from build123d import *

# Parameters (mm, degrees)
SKETCH1_W                      = 19
SKETCH1_H                      = 19
SKETCH1_R                      = 6.5
BOSS_EXTRUDE1_DEPTH            = 4
CUT_EXTRUDE1_REACH             = 16.018
SKETCH2_R                      = 1.5
CUT_EXTRUDE1_DIRECTION_2_REACH = 16.018
SKETCH5_W                      = 4
SKETCH5_H                      = 5
BOSS_EXTRUDE3_DEPTH            = 8
CUT_EXTRUDE2_REACH             = 22.31
SKETCH7_R                      = 1.5
CUT_EXTRUDE2_DIRECTION_2_REACH = 22.31


with BuildPart() as part:
    # Sketch1 → Boss-Extrude1 (new body)
    with BuildSketch(Plane.XY):
        Rectangle(SKETCH1_W, SKETCH1_H)
        Circle(SKETCH1_R, mode=Mode.SUBTRACT)
    extrude(amount=BOSS_EXTRUDE1_DEPTH)

    # Sketch2 → Cut-Extrude1 (cut, up to next)
    with BuildSketch(Plane(origin=(0, 0, 0), x_dir=(1, 0, 0), z_dir=(0, 1, 0)), mode=Mode.PRIVATE) as cut_extrude1_sk1:
        with Locations(Location((0, -2, 0), (0, 0, 90))):
            Circle(SKETCH2_R)
    cut_extrude1_tool1 = extrude(cut_extrude1_sk1.sketch, amount=CUT_EXTRUDE1_REACH, mode=Mode.PRIVATE) & part.part
    add(cut_extrude1_tool1.solids().sort_by_distance((0, 0, 2))[0], mode=Mode.SUBTRACT)

    # Sketch2 → Cut-Extrude1 direction 2 (cut, up to next)
    with BuildSketch(Plane(origin=(0, 0, 0), x_dir=(1, 0, 0), z_dir=(0, 1, 0)), mode=Mode.PRIVATE) as cut_extrude1_direction_2_sk1:
        with Locations(Location((0, -2, 0), (0, 0, 90))):
            Circle(SKETCH2_R)
    cut_extrude1_direction_2_tool1 = extrude(cut_extrude1_direction_2_sk1.sketch, amount=-CUT_EXTRUDE1_DIRECTION_2_REACH, mode=Mode.PRIVATE) & part.part
    add(cut_extrude1_direction_2_tool1.solids().sort_by_distance((0, 0, 2))[0], mode=Mode.SUBTRACT)

    # Sketch5 → Boss-Extrude3 (add)
    with BuildSketch(Plane.ZY.offset(9.5)):
        with Locations((2, 0)):
            Rectangle(SKETCH5_W, SKETCH5_H)
    extrude(amount=BOSS_EXTRUDE3_DEPTH)

    # Sketch7 → Cut-Extrude2 (cut, up to next)
    with BuildSketch(Plane(origin=(0, 0, 0), x_dir=(1, 0, 0), z_dir=(0, 1, 0)), mode=Mode.PRIVATE) as cut_extrude2_sk1:
        with Locations(Location((-15, -2, 0), (0, 0, 90))):
            Circle(SKETCH7_R)
    cut_extrude2_tool1 = extrude(cut_extrude2_sk1.sketch, amount=-CUT_EXTRUDE2_REACH, mode=Mode.PRIVATE) & part.part
    add(cut_extrude2_tool1.solids().sort_by_distance((-15, 0, 2))[0], mode=Mode.SUBTRACT)

    # Sketch7 → Cut-Extrude2 direction 2 (cut, up to next)
    with BuildSketch(Plane(origin=(0, 0, 0), x_dir=(1, 0, 0), z_dir=(0, 1, 0)), mode=Mode.PRIVATE) as cut_extrude2_direction_2_sk1:
        with Locations(Location((-15, -2, 0), (0, 0, 90))):
            Circle(SKETCH7_R)
    cut_extrude2_direction_2_tool1 = extrude(cut_extrude2_direction_2_sk1.sketch, amount=CUT_EXTRUDE2_DIRECTION_2_REACH, mode=Mode.PRIVATE) & part.part
    add(cut_extrude2_direction_2_tool1.solids().sort_by_distance((-15, 0, 2))[0], mode=Mode.SUBTRACT)


solid = part.part
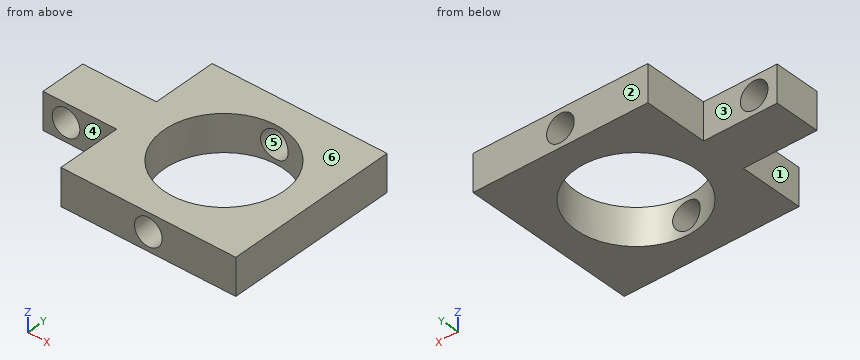
The model under review builds one solid part; all positions refer to its coordinate system, in mm. Face numbers are marked on the shaded views. A direction names the side the tool comes from. Give positions to 0.01 mm unless a question says otherwise; leave off trailing zeros. Loops run counter-clockwise (first coordinate to the right, second up) from the corner with the lowest first, then second, coordinate; pieces in that order, holes last. Notation, with made-up numbers: (-13, 76.25) -> (4, 76.25) arc R10 ccw to (4, 80.25) -> close; hole circle Ø11 at (81.5, 22). An arc over 180 degrees is marked (long way). Put each result on its own line as item: value. Start each with the question number.
1. We need section B-B on x = 0. State the section outline as (y, z) points, then the cut area to 3 significant figures.
2. Wall thickness on probe 1 along X at (y, z) = (-7.45, 2); probe 2 along Z at (x, y) = (-15, -1.35); probe 3 along X at (y, z) = (0.25, 3.1): over which ranges is each line inside the solid? List them lowest first.
3. For the marked faces 1, 2 and 3, list the 3-axis set-ups (+Z, -Z, +X, -X, +Y, -Y) from which the entire face can be reached by the end or side of a thin tool; tool diameter is ignored.
4. We need section D-D on x = -15. State the section outline as (y, z) points, then the cut area to 3 significant figures.
5. We need section A-A on y = 0. State the section outline as (x, z) points.
6. Mouldability with a two-part tool opening along Z and no side actions: class the marked faces 4, 5 and 6 as released by +Z, released by -Z, zero draft, split by the parting line, or undercut.
7. We need section C-C on z = 2. State the section outline as (x, y) points, then the cut area to 3 significant figures.
8. Clearance check with flat-ended pins moving along their axes: P1, Ø1.2, axis at y = -6, z = 1.5, coming from the -X side; P2, Ø2, axis at x = -13, z = 1, coming from the -Y side; P3, Ø1.2, axis at x = -14.5, z = 1, coming from the +Y side. State where each tip first meets the part, or that it passes through.
Determined:
1. outline: (-9.5, 0) -> (-6.5, 0) -> (-6.5, 0.5) -> (-9.5, 0.5) -> close; (-9.5, 3.5) -> (-6.5, 3.5) -> (-6.5, 4) -> (-9.5, 4) -> close; (6.5, 0) -> (9.5, 0) -> (9.5, 0.5) -> (6.5, 0.5) -> close; (6.5, 3.5) -> (9.5, 3.5) -> (9.5, 4) -> (6.5, 4) -> close
1. area: 6.00 mm^2
2. probe 1: -9.5 to -1.5, 1.5 to 9.5
2. probe 2: 0 to 0.5, 3.5 to 4
2. probe 3: -17.5 to -16.02, -13.98 to -6.5, 6.5 to 9.5
3. face 1: +Z, -Z, -X, -Y
3. face 2: +Z, -Z, +X, -X, +Y
3. face 3: +Z, -Z, -X, +Y
4. outline: (-2.5, 0) -> (2.5, 0) -> (2.5, 0.5) -> (-2.5, 0.5) -> close; (-2.5, 3.5) -> (2.5, 3.5) -> (2.5, 4) -> (-2.5, 4) -> close
4. area: 5.00 mm^2
5. outline: (-17.5, 0) -> (-6.5, 0) -> (-6.5, 4) -> (-17.5, 4) -> close; (6.5, 0) -> (9.5, 0) -> (9.5, 4) -> (6.5, 4) -> close; hole circle Ø3 at (-15, 2)
6. face 4: zero draft
6. face 5: undercut
6. face 6: released by +Z
7. outline: (-17.5, -2.5) -> (-16.5, -2.5) -> (-16.5, 2.5) -> (-17.5, 2.5) -> close; (-13.5, -2.5) -> (-9.5, -2.5) -> (-9.5, -9.5) -> (-1.5, -9.5) -> (-1.5, -6.32) arc R6.5 cw to (-1.5, 6.32) -> (-1.5, 9.5) -> (-9.5, 9.5) -> (-9.5, 2.5) -> (-13.5, 2.5) -> close; (1.5, -9.5) -> (9.5, -9.5) -> (9.5, 9.5) -> (1.5, 9.5) -> (1.5, 6.32) arc R6.5 cw to (1.5, -6.32) -> close
7. area: 235 mm^2
8. P1: x = -9.5
8. P2: y = -2.5
8. P3: y = 2.5
